Here's how the part is built. I have some questions about the finished solid (model axes, mm). Coordinates: 2 decimals unless noted, no trailing zeros. Write each loop counter-clockwise with the first axis right and the second up, starting at its lowest first coordinate (ties: lowest second). Pieces come first, ordered by that corner, then holes.
Item 1: Please list where these lines run through material, in increasing order: line 1 (Y direction, x = -88, z = 1.5); line 2 (X direction, y = 45, z = 2.5); line 3 (Y direction, x = -136, z = 1.45).
Item 2: If we mould it in two halves opening along Y, with no side actions, what happens to faces 1 (the face through (-144.32, -35.66, 1.57)), 2 (the face through (-77, 32, 0)), 3 (the face through (-34.12, 129.27, 1.57))? For each: pulls with the +Y half, pulls with the -Y half, needs draft (parallel to the pull), parting line crosses it, or undercut.
Item 3: I want a section at C-C (y = 68). Please give me the cut outline in (x, z) (3 decimals).
Item 4: I'm going to push a flat-ended pin straight in: P1, Ø1, axis at x = -14, z = 2, coming from the +Y side. Where does the tip first touch, or does it pass through?
Item 5: I want a section at A-A (x = -125). Please give me the cut outline in (y, z) (3 decimals), and give its area (3 significant figures).
Item 6: I want a section at D-D (z = 0.65). Count the separate pieces of the cut face and the enclosed holes in it, and give its area (3 significant figures).
Item 7: I want a section at B-B (x = -89.5). Please give me the cut outline in (y, z) (3 decimals), and give its area (3 significant figures).
from build123d import *

# Parameters (mm, degrees)
SKETCH1_R           = 6.477
SKETCH1_R_2         = 2.4
SKETCH1_R_3         = 10
SKETCH1_R_4         = 4.5000037
SKETCH1_R_5         = 2
BOSS_EXTRUDE1_DEPTH = 3.175


with BuildPart() as part:
    # Sketch1 → Boss-Extrude1 (new body)
    with BuildSketch(Plane.XY):
        with BuildLine():
            Line((-11.024299403, 39.940302972), (-16.104299403, 39.940302972))
            ThreePointArc((-16.104299403, 39.940302972), (-19.696401851, 41.428200524), (-21.184299403, 45.020302972))
            Line((-21.184299403, 45.020302972), (-21.184299403, 132.992318995))
            ThreePointArc((-21.184299403, 132.992318995), (-22.672196955, 136.584421443), (-26.264299403, 138.072318995))
            Line((-26.264299403, 138.072318995), (-140.691302272, 138.072318995))
            ThreePointArc((-140.691302272, 138.072318995), (-144.28340472, 136.584421443), (-145.771302272, 132.992318995))
            Line((-145.771302272, 132.992318995), (-145.771302272, -32.107679937))
            ThreePointArc((-145.771302272, -32.107679937), (-144.28340472, -35.699782385), (-140.691302272, -37.187679937))
            Line((-140.691302272, -37.187679937), (-11.024299403, -37.187679937))
            ThreePointArc((-11.024299403, -37.187679937), (-7.432196955, -35.699782385), (-5.944299403, -32.107679937))
            Line((-5.944299403, -32.107679937), (-5.944299403, 34.860302972))
            ThreePointArc((-5.944299403, 34.860302972), (-7.432196955, 38.452405421), (-11.024299403, 39.940302972))
        make_face()
        with Locations((-98.216033467, 50.891145684)):
            Circle(SKETCH1_R, mode=Mode.SUBTRACT)
        with Locations((-77.896041206, 50.908879471)):
            Circle(SKETCH1_R, mode=Mode.SUBTRACT)
        with Locations((-60.103647977, 50.875628534)):
            Circle(SKETCH1_R_2, mode=Mode.SUBTRACT)
        with Locations((-115.996026696, 50.875628621)):
            Circle(SKETCH1_R_2, mode=Mode.SUBTRACT)
        with Locations((-121.514302272, 31.820805424)):
            Circle(SKETCH1_R, mode=Mode.SUBTRACT)
        with Locations((-88.029366762, 95.350052781)):
            Circle(SKETCH1_R_3, mode=Mode.SUBTRACT)
        with Locations((-102.201189802, 83.458481295)):
            Circle(SKETCH1_R_4, mode=Mode.SUBTRACT)
        with Locations((-73.96362125, 107.367473015)):
            Circle(SKETCH1_R_4, mode=Mode.SUBTRACT)
        with Locations((-88.082707911, 6.449972374)):
            Circle(SKETCH1_R_3, mode=Mode.SUBTRACT)
        with Locations((-102.254530951, -5.441599113)):
            Circle(SKETCH1_R_4, mode=Mode.SUBTRACT)
        with Locations((-74.016962399, 18.467392607)):
            Circle(SKETCH1_R_4, mode=Mode.SUBTRACT)
        with Locations((-119.595565206, 129.182318995)):
            Circle(SKETCH1_R_5, mode=Mode.SUBTRACT)
        with Locations((-75.857800837, 129.182318995)):
            Circle(SKETCH1_R_5, mode=Mode.SUBTRACT)
        with Locations((-32.120036469, 129.182318995)):
            Circle(SKETCH1_R_5, mode=Mode.SUBTRACT)
        with Locations((-136.881302272, 110.132318995)):
            Circle(SKETCH1_R_5, mode=Mode.SUBTRACT)
        with Locations((-30.45529861, 114.196317591)):
            Circle(SKETCH1_R_5, mode=Mode.SUBTRACT)
        with Locations((-136.881302272, 50.442319529)):
            Circle(SKETCH1_R_5, mode=Mode.SUBTRACT)
        with Locations((-136.881302272, -9.247679937)):
            Circle(SKETCH1_R_5, mode=Mode.SUBTRACT)
        with Locations((-119.595565206, -28.297679937)):
            Circle(SKETCH1_R_5, mode=Mode.SUBTRACT)
        with Locations((-75.857800837, -28.297679937)):
            Circle(SKETCH1_R_5, mode=Mode.SUBTRACT)
        with Locations((-32.120036469, -28.297679937)):
            Circle(SKETCH1_R_5, mode=Mode.SUBTRACT)
        with Locations((-14.834299403, -9.247679937)):
            Circle(SKETCH1_R_5, mode=Mode.SUBTRACT)
        with Locations((-14.834299403, 31.050302972)):
            Circle(SKETCH1_R_5, mode=Mode.SUBTRACT)
    extrude(amount=BOSS_EXTRUDE1_DEPTH)


solid = part.part
Answer:
1. line 1: y = -37.19 to -3.55, 16.45 to 85.35, 105.35 to 138.07
1. line 2: x = -145.77 to -100.91, -95.52 to -80.55, -75.24 to -21.18
1. line 3: y = -37.19 to -11.04, -7.45 to 48.65, 52.24 to 108.34, 111.93 to 138.07
2. face 1: pulls with the -Y half
2. face 2: needs draft
2. face 3: undercut
3. outline: (-145.771, 0) - (-21.184, 0) - (-21.184, 3.175) - (-145.771, 3.175) - close
4. P1: stops at y = 39.94
5. outline: (-37.188, 0) - (26.362, 0) - (26.362, 3.175) - (-37.188, 3.175) - close; (37.28, 0) - (138.072, 0) - (138.072, 3.175) - (37.28, 3.175) - close
5. area: 522 mm2
6. separate pieces: 1
6. enclosed holes: 23
6. area: 21,500 mm2
7. outline: (-37.188, 0) - (-3.449, 0) - (-3.449, 3.175) - (-37.188, 3.175) - close; (16.349, 0) - (85.459, 0) - (85.459, 3.175) - (16.349, 3.175) - close; (105.241, 0) - (138.072, 0) - (138.072, 3.175) - (105.241, 3.175) - close
7. area: 431 mm2
